Geometry: final body of the model. Coordinates: model frame, mm. Face numbers are marked on the shaded views. A direction names the side the tool comes from. Coordinates: 2 decimals unless noted, no trailing zeros. Order: outer loops, then holes, each group sorted by start corner. A loop starts at its lowest first (then second) coordinate and runs counter-clockwise, first axis right, second up. Notation, with made-up numbers: M 22.25,71 L 35.25,71 A25 cw 35.25,92 Z; hole C 53,41.25 d1. An arc over 180 degrees is marked long. Write item = value, one per line.
from build123d import *

# Parameters (mm, degrees)
SKETCH1_W           = 50
SKETCH1_H           = 40
BOSS_EXTRUDE1_DEPTH = 20
SKETCH2_R           = 8
CUT_EXTRUDE1_DEPTH  = 43
SKETCH3_R           = 3
CUT_EXTRUDE2_DEPTH  = 43
SKETCH4_R           = 2.75
CUT_EXTRUDE3_DEPTH  = 50
SKETCH5_R           = 4.5
CUT_EXTRUDE4_DEPTH  = 6
CUT_EXTRUDE5_DEPTH  = 5


with BuildPart() as part:
    # Sketch1 → Boss-Extrude1 (new body)
    with BuildSketch(Plane.XY):
        with Locations((25, 20)):
            Rectangle(SKETCH1_W, SKETCH1_H)
    extrude(amount=BOSS_EXTRUDE1_DEPTH)

    # Sketch2 → Cut-Extrude1 (cut)
    with BuildSketch(Plane(origin=(0, 40, 0), x_dir=(1, 0, 0), z_dir=(0, 1, 0))):
        with Locations((25, -20)):
            Circle(SKETCH2_R)
    extrude(amount=-CUT_EXTRUDE1_DEPTH, mode=Mode.SUBTRACT)

    # Sketch3 → Cut-Extrude2 (cut)
    with BuildSketch(Plane.XY.offset(20)):
        with Locations((10, 30)):
            Circle(SKETCH3_R)
        with Locations((10, 10)):
            Circle(SKETCH3_R)
        with Locations((40, 30)):
            Circle(SKETCH3_R)
        with Locations((40, 10)):
            Circle(SKETCH3_R)
    extrude(amount=-CUT_EXTRUDE2_DEPTH, mode=Mode.SUBTRACT)

    # Sketch4 → Cut-Extrude3 (cut)
    with BuildSketch(Plane.XY.offset(20)):
        with Locations((10, 20)):
            Circle(SKETCH4_R)
        with Locations((40, 20)):
            Circle(SKETCH4_R)
    extrude(amount=-CUT_EXTRUDE3_DEPTH, mode=Mode.SUBTRACT)

    # Sketch5 → Cut-Extrude4 (cut)
    with BuildSketch(Plane.XY.offset(20)):
        with Locations((10, 20)):
            Circle(SKETCH5_R)
        with Locations((40, 20)):
            Circle(SKETCH5_R)
    extrude(amount=-CUT_EXTRUDE4_DEPTH, mode=Mode.SUBTRACT)

    # Sketch6 → Cut-Extrude5 (cut)
    with BuildSketch(Plane(origin=(0, 0, 0), x_dir=(-1, 0, 0), z_dir=(0, 0, -1))):
        Polygon((-3.937822174, 10), (-6.968911087, 15.25), (-13.031088913, 15.25), (-16.062177826, 10), (-13.031088913, 4.75), (-6.968911087, 4.75), align=None)
        Polygon((-43.031088913, 15.25), (-46.062177826, 10), (-43.031088913, 4.75), (-36.968911087, 4.75), (-33.937822174, 10), (-36.968911087, 15.25), align=None)
        Polygon((-36.968911087, 24.75), (-33.937822174, 30), (-36.968911087, 35.25), (-43.031088913, 35.25), (-46.062177826, 30), (-43.031088913, 24.75), align=None)
        Polygon((-6.968911087, 24.75), (-3.937822174, 30), (-6.968911087, 35.25), (-13.031088913, 35.25), (-16.062177826, 30), (-13.031088913, 24.75), align=None)
    extrude(amount=-CUT_EXTRUDE5_DEPTH, mode=Mode.SUBTRACT)


solid = part.part
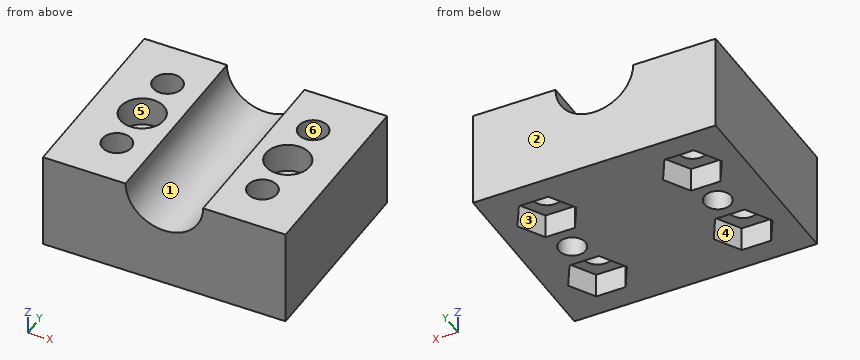
1) Section D-D, the plane z = 18.5. Return loops of the section in (x, y).
Numbers:
outline = M 0,0 L 17.14,0 L 17.14,40 L 0,40 Z; M 32.86,0 L 50,0 L 50,40 L 32.86,40 Z; hole C 10,20 d9; hole C 10,10 d6; hole C 10,30 d6; hole C 40,20 d9; hole C 40,10 d6; hole C 40,30 d6
2) Section A-A, the plane z = 8. Return loops of the section in (x, y).
Numbers:
outline = M 0,0 L 50,0 L 50,40 L 0,40 Z; hole C 10,10 d6; hole C 10,30 d6; hole C 10,20 d5.5; hole C 40,10 d6; hole C 40,30 d6; hole C 40,20 d5.5
3) Set-up query: the marked faces 4, 5 and 6. Return all of +Z, -Z, +X, -X, +Y, -Y with unobstructed straight access to the full face (end or side cutting, diameter ignored); none if empty.
Numbers:
face_4 = -Z
face_5 = +Z
face_6 = +Z, -Z
4) Section B-B, the plane x = 10. Return loops of the section in (y, z), and give its area (3 significant figures).
Numbers:
outline = M 0,0 L 4.75,0 L 4.75,5 L 7,5 L 7,20 L 0,20 Z; M 13,5 L 15.25,5 L 15.25,0 L 17.25,0 L 17.25,14 L 15.5,14 L 15.5,20 L 13,20 Z; M 22.75,0 L 24.75,0 L 24.75,5 L 27,5 L 27,20 L 24.5,20 L 24.5,14 L 22.75,14 Z; M 33,5 L 35.25,5 L 35.25,0 L 40,0 L 40,20 L 33,20 Z
area = 384 mm²
5) Pin query (flat end, axial travel): pin 1 (8 mm diameter, centred on x = 40, y = 30, fed in from -Z). Return the tip coordinate at first contact, or that it passes through.
Numbers:
pin_1 = 5
6) Section C-C, the plane y = 20. Return loops of the section in (x, z).
Numbers:
outline = M 0,0 L 7.25,0 L 7.25,14 L 5.5,14 L 5.5,20 L 0,20 Z; M 12.75,0 L 37.25,0 L 37.25,14 L 35.5,14 L 35.5,20 L 33,20 A8 cw 17,20 L 14.5,20 L 14.5,14 L 12.75,14 Z; M 42.75,0 L 50,0 L 50,20 L 44.5,20 L 44.5,14 L 42.75,14 Z
7) Line query: L1, parallel to Y at x = 10, z = 12; L2, parallel to Y at x = 40, z = 14.75; L3, parallel to X at y = 11, z = 7.5. Output: solid intervals per line, ascending.
Numbers:
L1 = 0 to 7, 13 to 17.25, 22.75 to 27, 33 to 40
L2 = 0 to 7, 13 to 15.5, 24.5 to 27, 33 to 40
L3 = 0 to 7.17, 12.83 to 37.17, 42.83 to 50
8) Mould query, pull axis Y, two halves, no side actions, for the marked faces 1, 2 and 3. Classes: pulls with the +Y half, pulls with the -Y half, needs draft (parallel to the pull), parting line crosses it, or undercut.
Numbers:
face_1 = needs draft
face_2 = pulls with the +Y half
face_3 = undercut
